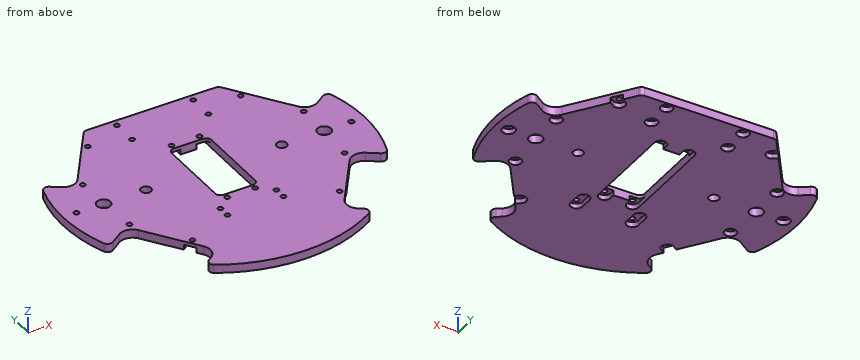
```python
from build123d import *

# Parameters (mm, degrees)
SKETCH_1_R                  = 89
EXTRUDE_1_DEPTH             = 5
HOLE_WIZARD_8_D             = 3
HOLE_WIZARD_8_CBORE_D       = 7
HOLE_WIZARD_8_CBORE_DEPTH   = 3
CUT_EXTRUDE_2_DEPTH         = 10
CUT_EXTRUDE_3_DEPTH         = 10
HOLE_WIZARD_8_2_D           = 3
HOLE_WIZARD_8_2_CBORE_D     = 7
HOLE_WIZARD_8_2_CBORE_DEPTH = 3
SKETCH_27_W                 = 23.5
SKETCH_27_H                 = 49.1
CUT_EXTRUDE_4_DEPTH         = 10
FILLET_1_R                  = 3
HOLE_WIZARD_1_0_1_1_D       = 3
FILLET_2_DEPTH              = 5
FILLET_START                = 3
FILLET_2_2_DEPTH            = 2
CUT_EXTRUDE_8_DEPTH         = 3
CUT_EXTRUDE_11_DEPTH        = 3
CUT_EXTRUDE_9_DEPTH         = 3
HOLE_WIZARD_8_3_D           = 3.2
HOLE_WIZARD_8_3_CBORE_D     = 7.5
HOLE_WIZARD_8_3_CBORE_DEPTH = 3
SKETCH_50_R                 = 3
SKETCH_50_R_2               = 4
CUT_EXTRUDE_10_DEPTH        = 126.964280651


with BuildPart() as part:
    # 草图1 → 拉伸1 (new body)
    with BuildSketch(Plane.XY):
        Circle(SKETCH_1_R)
    extrude(amount=EXTRUDE_1_DEPTH)

    # Hole Wizard 8 (through all)
    with Locations(Plane(origin=(45.056156837, 48.977181137, 0), x_dir=(-1, 0, 0), z_dir=(0, 0, -1))):
        with Locations((0, 0), (-20.075175273, -28.67032155), (1.720729309, -100.411818407), (-18.354445964, -71.741496856)):
            hole_wizard_8 = CounterBoreHole(HOLE_WIZARD_8_D / 2, HOLE_WIZARD_8_CBORE_D / 2, HOLE_WIZARD_8_CBORE_DEPTH)

    # 镜向6: Hole Wizard 8 across plane
    add(hole_wizard_8.mirror(Plane(origin=(0, 0, 0), x_dir=(0, 0, 1), z_dir=(1, 0, 0))), mode=Mode.SUBTRACT)

    # 草图21 → Cut-Extrude 2 (cut)
    with BuildSketch(Plane(origin=(0, 0, 0), x_dir=(-1, 0, 0), z_dir=(0, 0, -1))):
        with BuildLine():
            Line((-39.599804667, 62), (39.599804667, 62))
            Line((39.599804667, 62), (69.309517552, 19.570132763))
            Line((69.309517552, 19.570132763), (83.87400404, 29.768295992))
            ThreePointArc((83.87400404, 29.768295992), (0, 89), (-83.87400404, 29.768295992))
            Line((-83.87400404, 29.768295992), (-69.309517552, 19.570132763))
            Line((-69.309517552, 19.570132763), (-39.599804667, 62))
        make_face()
    extrude(amount=-CUT_EXTRUDE_2_DEPTH, mode=Mode.SUBTRACT)

    # 草图22 → Cut-Extrude 3 (cut)
    with BuildSketch(Plane(origin=(0, 0, 0), x_dir=(-1, 0, 0), z_dir=(0, 0, -1))):
        with BuildLine():
            Line((-82.012277652, -34.568574085), (-66.44163537, -23.665892984))
            Line((-66.44163537, -23.665892984), (-37.189237116, -65.442647243))
            Line((-37.189237116, -65.442647243), (-49.428242542, -74.012491103))
            ThreePointArc((-49.428242542, -74.012491103), (-68.615655901, -56.682376144), (-82.012277652, -34.568574085))
        make_face()
    cut_extrude_3 = extrude(amount=-CUT_EXTRUDE_3_DEPTH, mode=Mode.SUBTRACT)

    # 镜向7: Cut-Extrude 3 across plane
    add(cut_extrude_3.mirror(Plane(origin=(0, 0, 0), x_dir=(0, 0, 1), z_dir=(1, 0, 0))), mode=Mode.SUBTRACT)

    # Hole Wizard 8 2 (through all)
    with Locations(Plane(origin=(22.5, 58, 0), x_dir=(-1, 0, 0), z_dir=(0, 0, -1))):
        with Locations((0, 0), (0, -15), (45, -15), (45, 0), (-127.702769625, 168.922663635)):
            CounterBoreHole(HOLE_WIZARD_8_2_D / 2, HOLE_WIZARD_8_2_CBORE_D / 2, HOLE_WIZARD_8_2_CBORE_DEPTH)

    # 草图27 → Cut-Extrude 4 (cut)
    with BuildSketch(Plane(origin=(0, 0, 0), x_dir=(-1, 0, 0), z_dir=(0, 0, -1))):
        with Locations((0, 0.5)):
            Rectangle(SKETCH_27_W, SKETCH_27_H)
    extrude(amount=-CUT_EXTRUDE_4_DEPTH, mode=Mode.SUBTRACT)

    # 圆角1
    fillet_1_edges = [part.edges().sort_by_distance(p)[0] for p in [
        (82.012277652, -34.568574085, 2.5),
        (49.428242542, -74.012491103, 2.5),
        (-82.012277652, -34.568574085, 2.5),
        (-49.428242542, -74.012491103, 2.5),
        (11.75, -24.05, 2.5),
        (11.75, 25.05, 2.5),
        (-11.75, 25.05, 2.5),
        (-11.75, -24.05, 2.5),
        (39.599804667, 62, 2.5),
        (83.87400404, 29.768295992, 2.5),
        (-83.87400404, 29.768295992, 2.5),
        (-39.599804667, 62, 2.5),
    ]]
    fillet(fillet_1_edges, radius=FILLET_1_R)

    # Ø1.0 (1) 直径孔1 (through all)
    with Locations(Plane(origin=(8.25, 28, 0), x_dir=(-1, 0, 0), z_dir=(0, 0, -1))):
        with Locations((0, 0), (16.5, 0), (-8.25, -62), (24.75, -62), (0, -55), (16.5, -55), (-8.25, -69), (24.75, -69)):
            Hole(HOLE_WIZARD_1_0_1_1_D / 2)

    # 圆角2: read off the stored shape, not the designer's step
    # 圆角2 outline → 圆角2 (add)
    with BuildSketch(Plane.XY):
        with BuildLine():
            Line((-37.189237116, -65.442647243), (-41.491060389, -59.299006911))
            ThreePointArc((-41.491060389, -59.299006911), (-40.248642573, -64.903191516), (-43.332877448, -69.744470516))
            Line((-43.332877448, -69.744470516), (-37.189237116, -65.442647243))
        make_face()
        with BuildLine():
            ThreePointArc((-64.834029308, -25.961792377), (-66.003394893, -25.115364244), (-66.73169872, -23.868997528))
            Line((-66.73169872, -23.868997528), (-72.585275702, -27.967716257))
            ThreePointArc((-72.585275702, -27.967716257), (-66.981091097, -26.725298441), (-62.139812097, -29.809533316))
            Line((-62.139812097, -29.809533316), (-64.834029308, -25.961792377))
        make_face()
        with BuildLine():
            ThreePointArc((-68.622817869, 20.550841547), (-67.998364265, 22.314377114), (-66.554758617, 23.504336245))
            Line((-66.554758617, 23.504336245), (-65.007694279, 25.713773095))
            ThreePointArc((-65.007694279, 25.713773095), (-69.848973279, 22.62953822), (-75.453157884, 23.871956035))
            Line((-75.453157884, 23.871956035), (-69.309517552, 19.570132763))
            Line((-69.309517552, 19.570132763), (-68.622817869, 20.550841547))
        make_face()
        with BuildLine():
            ThreePointArc((75.453157884, 23.871956035), (69.848973279, 22.62953822), (65.007694279, 25.713773095))
            Line((65.007694279, 25.713773095), (66.554758617, 23.504336245))
            ThreePointArc((66.554758617, 23.504336245), (67.998364265, 22.314377114), (68.622817869, 20.550841547))
            Line((68.622817869, 20.550841547), (69.309517552, 19.570132763))
            Line((69.309517552, 19.570132763), (75.453157884, 23.871956035))
        make_face()
        with BuildLine():
            ThreePointArc((43.332877448, -69.744470516), (40.248642573, -64.903191516), (41.491060389, -59.299006911))
            Line((41.491060389, -59.299006911), (37.189237116, -65.442647243))
            Line((37.189237116, -65.442647243), (43.332877448, -69.744470516))
        make_face()
        with BuildLine():
            ThreePointArc((62.139812097, -29.809533316), (66.981091097, -26.725298441), (72.585275702, -27.967716257))
            Line((72.585275702, -27.967716257), (66.73169872, -23.868997528))
            ThreePointArc((66.73169872, -23.868997528), (66.003394893, -25.115364244), (64.834029308, -25.961792377))
            Line((64.834029308, -25.961792377), (62.139812097, -29.809533316))
        make_face()
    extrude(amount=FILLET_2_DEPTH)

    # Fillet 2 2 outline → Fillet 2 2 (add)
    with BuildSketch(Plane.XY.offset(FILLET_START)):
        with BuildLine():
            Line((-66.44163537, -23.665892984), (-66.73169872, -23.868997528))
            ThreePointArc((-66.73169872, -23.868997528), (-66.003394893, -25.115364244), (-64.834029308, -25.961792377))
            Line((-64.834029308, -25.961792377), (-66.44163537, -23.665892984))
        make_face()
        with BuildLine():
            Line((-68.622817869, 20.550841547), (-66.554758617, 23.504336245))
            ThreePointArc((-66.554758617, 23.504336245), (-67.998364265, 22.314377114), (-68.622817869, 20.550841547))
        make_face()
        with BuildLine():
            ThreePointArc((68.622817869, 20.550841547), (67.998364265, 22.314377114), (66.554758617, 23.504336245))
            Line((66.554758617, 23.504336245), (68.622817869, 20.550841547))
        make_face()
        with BuildLine():
            ThreePointArc((64.834029308, -25.961792377), (66.003394893, -25.115364244), (66.73169872, -23.868997528))
            Line((66.73169872, -23.868997528), (66.44163537, -23.665892984))
            Line((66.44163537, -23.665892984), (64.834029308, -25.961792377))
        make_face()
    extrude(amount=FILLET_2_2_DEPTH)

    # 草图46 → 切除-拉伸8 (cut)
    with BuildSketch(Plane(origin=(0, 0, 0), x_dir=(-1, 0, 0), z_dir=(0, 0, -1))):
        with BuildLine():
            Line((-4.75, 28), (-4.75, -27))
            ThreePointArc((-4.75, -27), (-8.25, -30.5), (-11.75, -27))
            Line((-11.75, -27), (-11.75, 28))
            ThreePointArc((-11.75, 28), (-8.25, 31.5), (-4.75, 28))
        make_face()
        with BuildLine():
            Line((11.75, 28), (11.75, -27))
            ThreePointArc((11.75, -27), (8.25, -30.5), (4.75, -27))
            Line((4.75, -27), (4.75, 28))
            ThreePointArc((4.75, 28), (8.25, 31.5), (11.75, 28))
        make_face()
    extrude(amount=-CUT_EXTRUDE_8_DEPTH, mode=Mode.SUBTRACT)

    # 草图51 → 切除-拉伸11 (cut)
    with BuildSketch(Plane(origin=(0, 0, 0), x_dir=(-1, 0, 0), z_dir=(0, 0, -1))):
        with BuildLine():
            Line((-13, -34), (-13, -41))
            ThreePointArc((-13, -41), (-16.5, -44.5), (-20, -41))
            Line((-20, -41), (-20, -34))
            ThreePointArc((-20, -34), (-16.5, -30.5), (-13, -34))
        make_face()
    cut_extrude_11 = extrude(amount=-CUT_EXTRUDE_11_DEPTH, mode=Mode.SUBTRACT)

    # 镜向8: 切除-拉伸11 across plane
    add(cut_extrude_11.mirror(Plane(origin=(0, 0, 0), x_dir=(0, 0, 1), z_dir=(1, 0, 0))), mode=Mode.SUBTRACT)

    # 草图47 → 切除-拉伸9 (cut)
    with BuildSketch(Plane(origin=(0, 0, 0), x_dir=(-1, 0, 0), z_dir=(0, 0, -1))):
        with BuildLine():
            Line((-41.327910001, -54.301669425), (-43.785366134, -56.022398734))
            ThreePointArc((-43.785366134, -56.022398734), (-48.659915816, -55.162884106), (-47.800401188, -50.288334424))
            Line((-47.800401188, -50.288334424), (-45.342945056, -48.567605115))
            ThreePointArc((-45.342945056, -48.567605115), (-40.468395373, -49.427119742), (-41.327910001, -54.301669425))
        make_face()
        with BuildLine():
            Line((-47.063674365, 46.110148982), (-49.521130497, 47.830878291))
            ThreePointArc((-49.521130497, 47.830878291), (-50.380645125, 52.705427973), (-45.506095443, 53.564942601))
            Line((-45.506095443, 53.564942601), (-43.04863931, 51.844213292))
            ThreePointArc((-43.04863931, 51.844213292), (-42.189124682, 46.969663609), (-47.063674365, 46.110148982))
        make_face()
        with BuildLine():
            Line((43.04863931, 51.844213292), (45.506095443, 53.564942601))
            ThreePointArc((45.506095443, 53.564942601), (50.380645125, 52.705427973), (49.521130497, 47.830878291))
            Line((49.521130497, 47.830878291), (47.063674365, 46.110148982))
            ThreePointArc((47.063674365, 46.110148982), (42.189124682, 46.969663609), (43.04863931, 51.844213292))
        make_face()
        with BuildLine():
            Line((45.342945056, -48.567605115), (47.800401188, -50.288334424))
            ThreePointArc((47.800401188, -50.288334424), (48.659915816, -55.162884106), (43.785366134, -56.022398734))
            Line((43.785366134, -56.022398734), (41.327910001, -54.301669425))
            ThreePointArc((41.327910001, -54.301669425), (40.468395373, -49.427119742), (45.342945056, -48.567605115))
        make_face()
    extrude(amount=-CUT_EXTRUDE_9_DEPTH, mode=Mode.SUBTRACT)

    # Hole Wizard 8 3 (through all)
    with Locations(Plane(origin=(81, 0, 0), x_dir=(-1, 0, 0), z_dir=(0, 0, -1))):
        with Locations((0, 0), (162, 0)):
            CounterBoreHole(HOLE_WIZARD_8_3_D / 2, HOLE_WIZARD_8_3_CBORE_D / 2, HOLE_WIZARD_8_3_CBORE_DEPTH)

    # 草图50 → 切除-拉伸10 (cut, through all)
    with BuildSketch(Plane(origin=(0, 0, 0), x_dir=(-1, 0, 0), z_dir=(0, 0, -1))):
        with Locations((-40.001582071, 0)):
            Circle(SKETCH_50_R)
        with Locations((40, 0)):
            Circle(SKETCH_50_R)
        with Locations((-65, 0)):
            Circle(SKETCH_50_R_2)
        with Locations((65, 0)):
            Circle(SKETCH_50_R_2)
    extrude(amount=-CUT_EXTRUDE_10_DEPTH, mode=Mode.SUBTRACT)


solid = part.part
```
The model under review builds one solid part; all positions refer to its coordinate system, in mm. Round coordinates to 2 decimals unless told otherwise and drop trailing zeros. Write each question's results on one line, items separated by ' | '. Start each with the question number.
Q1. Take a section at A-A on z = 0.95. Give the number of separate pieces and of enclosed holes in the cut face, plus the area to 3 significant figures.
Q2. Wall thickness on line 1 along Y through (x, z) = (1, 1.85); line 2 along X through (y, z) = (42, 4.2); line 3 along X through (y, z) = (-25.5, 2.2): over which ranges is each line inside the solid? List them lowest first. Write a range as [from, to].
Q3. Insertion check: P1, Ø6.5, axis at x = -22.5, y = 43, coming from the +Z side; P2, Ø1.9, axis at x = 81, y = 0, coming from the -Z side; P3, Ø1, axis at y = -67, z = 2.5, coming from the -X side; P4, Ø3.5, axis at x = 45.06, y = 48.98, coming from the -Z side. Each pin has a flat end and moves straight along its axis. Give the tip position at first contact, or say it passes through.
Data:
1) separate pieces: 1 | enclosed holes: 17 | area: 16,600 mm²
2) line 1: y = [-88.99, -24.05], [25.05, 62] | line 2: x = [-53.6, -23.62], [-21.38, 21.38], [23.62, 53.6] | line 3: x = [-85.27, -65.59], [-61.23, -11.75], [-4.75, 4.75], [11.75, 61.23], [65.59, 85.27]
3) P1: stops at z = 5 | P2: passes through | P3: stops at x = -41.23 | P4: stops at z = 3
